Model file for the job. Use its own axes, mm. A direction names the side the tool comes from. Give positions to 0.01 mm unless a question says otherwise; leave off trailing zeros. Loops run counter-clockwise (first coordinate to the right, second up) from the corner with the lowest first, then second, coordinate; pieces in that order, holes last. Notation, with made-up numbers: M 57,-25.5 L 86,-25.5 A28 ccw 86,-0.5 Z; hole C 13,72.5 d8. An arc over 180 degrees is marked long. Answer in a Markdown table with one row per item.
Autodesk Inventor part; units mm, degrees
ref_plane "YZ Plane" through (0, 0, 0) normal (1, 0, 0) x (0, 1, 0)
ref_plane "XZ Plane" through (0, 0, 0) normal (0, 1, 0) x (-1, 0, 0)
ref_plane "XY Plane" through (0, 0, 0) normal (0, 0, 1) x (1, 0, 0)
sketch "Szkic10" plane through (0, 0, 0) normal (0, 1, 0) x (-1, 0, 0)
  line L0 (-25, 60) -> (25, 60)
  line L1 (25, 60) -> (25, -60)
  line L2 (25, -60) -> (-25, -60)
  line L3 (-25, -60) -> (-25, 60)
  line L4 (-25, 60) -> (25, -60) construction
  line L5 (25, 60) -> (-25, -60) construction
  point P0 (0, 0)
  dimension "d75" = 50
  dimension "d76" = 120
extrude "Wyciągnięcie proste6" add sketch "Szkic10" along normal blind 10
sketch "Szkic11" plane through (-25, 0, -60) normal (-1, 0, 0) x (0, 0, 1)
  line L0 (120, 0) -> (0, 0)
  line L1 (120, 0) -> (120, 10)
  line L2 (0, 10) -> (120, 10)
  line L3 (0, 0) -> (0, 10)
  line L4 (0, 0) -> (120, 0)
  line L5 (0, 0) -> (0, 5)
  line L6 (0, 5) -> (120, 5)
  line L7 (0, 5) -> (20, 5)
  line L8 (20, 5) -> (40, 5)
  line L9 (40, 5) -> (80, 5)
  line L10 (80, 5) -> (100, 5)
  circle A0 centre (20, 5) radius 2.5
  circle A1 centre (40, 5) radius 2.5
  circle A2 centre (80, 5) radius 2.5
  circle A3 centre (100, 5) radius 2.5
  point P0 (60, 0)
  dimension "d79" = 5
  dimension "d80" = 20
  dimension "d81" = 20
  dimension "d84" = 5
  dimension "d85" = 5
  dimension "d86" = 5
  dimension "d87" = 5
  dimension "d105" = 20
  dimension "d106" = 20
extrude "Wyciągnięcie proste7" cut sketch "Szkic11" against normal blind 20 contours A3 L6 | L6 A3 | A0 L6 | L6 A0 | A2 L6 | L6 A2 | A1 L6 | L6 A1
sketch "Szkic12" plane through (0, 10, 0) normal (0, 1, 0) x (1, 0, 0)
  line L0 (25, -60) -> (25, 60)
  line L1 (25, 0) -> (3, 0)
  circle A0 centre (3, 0) radius 13
  point P0 (0, 0)
  dimension "d102" = 22
  dimension "d103" = 26
extrude "Wyciągnięcie proste8" cut sketch "Szkic12" against normal up to next
sketch "Szkic13" plane through (0, 0, 0) normal (0, -1, 0) x (1, 0, 0)
  line L0 (25, 60) -> (-25, 60)
  line L1 (-25, 60) -> (-25, -60)
  line L2 (-25, -60) -> (25, -60)
  line L3 (25, -60) -> (25, 60)
  line L4 (25, 60) -> (25, 50)
  line L5 (25, -60) -> (25, 60)
  line L6 (25, 50) -> (-25, 50)
  line L7 (25, -60) -> (25, -50)
  line L8 (25, -50) -> (-25, -50)
  line L9 (25, 50) -> (15, 50)
  line L10 (25, -50) -> (15, -50)
  circle A0 centre (15, 50) radius 5
  circle A1 centre (15, -50) radius 5
  point P0 (0, 0)
  dimension "d93" = 10
  dimension "d94" = 10
  dimension "d95" = 10
  dimension "d96" = 10
  dimension "d97" = 10
  dimension "d98" = 10
extrude "Wyciągnięcie proste9" cut sketch "Szkic13" against normal blind 3 contours A0 L6 | L6 A0 | A1 L8 | L8 A1
sketch "Szkic14" plane through (15, 3, -50) normal (0, -1, 0) x (1, 0, 0)
  circle A0 centre (0, 0) radius 5
  circle A1 centre (0, 100) radius 5
  point P0 (-15, 50)
extrude "Wyciągnięcie proste10" cut sketch "Szkic14" against normal blind 10
sketch "Szkic15" plane through (25, 0, 60) normal (1, 0, 0) x (0, 0, -1)
  line L0 (120, 0) -> (0, 0)
  line L1 (120, 0) -> (120, 10)
  line L2 (0, 10) -> (120, 10)
  line L3 (0, 0) -> (0, 10)
  point P0 (60, 0)
extrude "Wyciągnięcie proste11" add sketch "Szkic15" along normal blind 7
sketch "Szkic16" plane through (-25, 0, 60) normal (0, 0, 1) x (1, 0, 0)
  line L0 (57, 0) -> (0, 0)
  line L1 (57, 10) -> (57, 0)
  line L2 (0, 10) -> (57, 10)
  line L3 (0, 0) -> (0, 10)
  line L4 (35, 10) -> (45, 10)
  line L5 (45, 0) -> (35, 0)
  line L6 (53, 0) -> (45, 0)
  line L7 (57, 0) -> (0, 0)
  line L8 (45, 0) -> (45, 10)
  line L9 (0, 10) -> (57, 10)
  line L10 (57, 10) -> (57, 0)
  line L11 (53, 5) -> (45, 5)
  line L12 (45, 5) -> (49, 5)
  circle A0 centre (49, 5) radius 2
  line L13 (49, 5) -> (53, 5)
  line L14 (53, 5) -> (53, 10)
  line L15 (53, 5) -> (53, 0)
  point P0 (25, 0)
  dimension "d113" = 4
  dimension "d114" = 4
  dimension "d115" = 5
  dimension "d116" = 45
  dimension "d117" = 4
sketch "Szkic17" plane through (-25, 0, -60) normal (0, 0, -1) x (-1, 0, 0)
  line L0 (-53, 10) -> (0, 10)
  line L1 (-53, 0) -> (-53, 10)
  line L2 (0, 0) -> (-53, 0)
  line L3 (0, 10) -> (0, 0)
  line L4 (-35, 0) -> (-45, 0)
  line L5 (-45, 10) -> (-35, 10)
  line L6 (-53, 10) -> (-45, 10)
  line L7 (-53, 10) -> (0, 10)
  line L8 (-45, 10) -> (-45, 0)
  line L9 (0, 0) -> (-53, 0)
  line L10 (-53, 0) -> (-53, 10)
  line L11 (-53, 5) -> (-45, 5)
  line L12 (-45, 5) -> (-49, 5)
  circle A0 centre (-49, 5) radius 2
  line L13 (-49, 5) -> (-53, 5)
  line L14 (-53, 5) -> (-53, 0)
  line L15 (-53, 5) -> (-53, 10)
  line L16 (0, 0) -> (-57, 0)
  line L17 (0, 0) -> (0, 10)
  point P0 (-25, 0)
  point P1 (-25, 10)
  dimension "d119" = 4
  dimension "d120" = 4
  dimension "d121" = 5
  dimension "d122" = 45
  dimension "d123" = 4
hole "Otwór4" at (24, 5, -60) direction (0, 0, 1) diameter 4 depth 20 tip angle 118
hole "Otwór5" at (24, 5, 60) direction (0, 0, -1) diameter 4 depth 20 tip angle 118
sketch "Szkic18" plane through (0, 0, 0) normal (0, -1, 0) x (1, 0, 0)
  circle A0 centre (15, -50) radius 5
  circle A1 centre (15, 50) radius 5
  circle A2 centre (3, 0) radius 13
  line L0 (32, 60) -> (-25, 60)
  line L1 (-25, 60) -> (-25, -60)
  line L2 (-25, -60) -> (32, -60)
  line L3 (32, 60) -> (32, -60)
  line L4 (15, -50) -> (32, -50)
  line L5 (15, 50) -> (32, 50)
  line L6 (32, -60) -> (32, 60)
  line L7 (15, 50) -> (15, 51.5)
  line L8 (15, 51.5) -> (32, 51.5)
  line L9 (15, 50) -> (15, 48.5)
  line L10 (15, 48.5) -> (32, 48.5)
  line L11 (15, -50) -> (15, -48.5)
  line L12 (15, -48.5) -> (32, -48.5)
  line L13 (15, -50) -> (15, -51.5)
  line L14 (15, -51.5) -> (32, -51.5)
  point P0 (0, 0)
  dimension "d138" = 1.5
  dimension "d139" = 1.5
  dimension "d140" = 1.5
  dimension "d141" = 1.5
extrude "Wyciągnięcie proste12" cut sketch "Szkic18" against normal up to next contours L4 L11 L12 A0 | L4 L3 L14 A0 | A0 L14 L13 L4 | A0 L12 L3 L4 | L10 A1 L5 L3 | L5 A1 L8 L3 | L10 L9 L5 A1 | L5 L7 L8 A1
thread "Gwint9"
thread "Gwint10"
thread "Gwint11"
thread "Gwint12"
sketch "Szkic20" plane through (0, 0, 0) normal (0, -1, 0) x (1, 0, 0)
  line L0 (32, 48.5) -> (32, -48.5)
  line L1 (-25, 60) -> (-25, -60)
  circle A0 centre (3, 0) radius 13
  circle A1 centre (22, 16) radius 2.5
  circle A2 centre (22, -16) radius 2.5
  circle A3 centre (-18.5, 0) radius 2.5
  circle A4 centre (3, 0) radius 15
  line L2 (-25, 25) -> (-25, -25)
  line L3 (-25, -25) -> (32, -25)
  line L4 (32, -25) -> (32, 25)
  line L5 (32, 25) -> (-25, 25)
  point P0 (0, 0)
extrude "Wyciągnięcie proste14" cut sketch "Szkic20" against normal up to next contours A1 | A2 | A3
thread "Gwint13"
thread "Gwint14"
thread "Gwint15"
sketch "Szkic21" plane through (0, 10, 0) normal (0, 1, 0) x (1, 0, 0)
  line L0 (32, 48.5) -> (32, -48.5)
  line L1 (32, -51.5) -> (32, -60)
  line L2 (32, 60) -> (32, 30)
  line L3 (-25, -60) -> (-25, 60)
  line L4 (-25, -60) -> (32, -60)
  line L5 (-25, 60) -> (32, 60)
  circle A0 centre (0, 50) radius 2.5
  circle A1 centre (-20, 30) radius 2.5
  circle A2 centre (-20, -30) radius 2.5
  circle A3 centre (0, -50) radius 2.5
  line L6 (-25, -60) -> (32, -60)
  line L7 (32, -51.5) -> (32, -60)
  point P0 (0, 0)
extrude "Wyciągnięcie proste15" cut sketch "Szkic21" against normal up to next
thread "Gwint16"
thread "Gwint17"
thread "Gwint18"
thread "Gwint19"
properties part number "Podstawa górna osi Z"
Q1. Drop flat-ended pins along their axis: pin 1 (2.5 mm diameter, centred on x = 24, y = 5, fed in from +Z); pin 2 (3.5 mm diameter, centred on x = 24, y = 5, fed in from +Z); pin 3 (2.5 mm diameter, centred on y = 5, z = 39, fed in from -X); pin 4 (4.5 mm diameter, centred on x = -18.5, z = 0, fed in from -Y). Give the stop position or say it passes through.
Reported:
| item | result |
|---|---|
| pin 1 | z = 39.55 |
| pin 2 | z = 39.85 |
| pin 3 | x = -5 |
| pin 4 | through |
Q2. 3-axis set-ups, long thin cutter, end or side, ignore diameter. For faces 1 (the face through (3, 5, 60)), 2 (the face through (22.648, 6.474, 44.19)), 3 (the face through (24, 3, -44)), 4 (the face through (-5, 5, 20)), 5 (the face through (26, 4, -48.5)): which of +Z, -Z, +X, -X, +Y, -Y reach the whole face in a straight line?
Reported:
| item | result |
|---|---|
| face 1 | +Z, +X, -X, +Y, -Y |
| face 2 | +Z |
| face 3 | -Z |
| face 4 | -X |
| face 5 | +X, +Y, -Y |
Q3. Saw through at A-A (z = 30). Give the cut face in (x, y), and give its area (3 significant figures).
Reported:
| item | result |
|---|---|
| outline | M -25,0 L -22.5,0 L -22.5,10 L -25,10 Z; M -17.5,0 L 32,0 L 32,10 L -17.5,10 Z |
| area | 520 mm² |
Q4. Probe probe 1 along Z at (x, y) = (22, 2.5); probe 2 along Y at (x, z) = (-19.75, -20); probe 3 along Z at (x, y) = (29, 9.25). List the from-to ranges inside material, lowest first.
Reported:
| item | result |
|---|---|
| probe 1 | -60 to -51.5, -48.5 to -18.5, -13.5 to 13.5, 18.5 to 48.5, 51.5 to 60 |
| probe 2 | 0 to 2.5, 7.5 to 10 |
| probe 3 | -60 to -51.5, -48.5 to 48.5, 51.5 to 60 |
Q5. Saw through at D-D (z = 50). Give the cut face in (x, y).
Reported:
| item | result |
|---|---|
| outline | M -25,0 L -2.5,0 L -2.5,10 L -25,10 Z; M 2.5,0 L 10,0 L 10,10 L 2.5,10 Z |
Q6. Mould opens along X. For faces 6 (the face through (-5, 5, -40)), 7 (the face through (3, 5, -60)), 8 (the face through (24.235, 4.744, -39.007)) say: released by +X, released by -X, zero draft, split by the parting line, or undercut.
Reported:
| item | result |
|---|---|
| face 6 | released by -X |
| face 7 | zero draft |
| face 8 | undercut |
Q7. Saw through at B-B (x = -7). Give the cut face in (y, z).
Reported:
| item | result |
|---|---|
| outline | M 0,-60 L 10,-60 L 10,-8.31 L 0,-8.31 Z; M 0,8.31 L 10,8.31 L 10,60 L 0,60 Z; hole C 5,-40 d5; hole C 5,-20 d5; hole C 5,20 d5; hole C 5,40 d5 |
Q8. Saw through at C-C (x = 0). Give the cut face in (y, z), and give its area (3 significant figures).
Reported:
| item | result |
|---|---|
| outline | M 0,-60 L 10,-60 L 10,-52.5 L 0,-52.5 Z; M 0,-47.5 L 10,-47.5 L 10,-12.65 L 0,-12.65 Z; M 0,12.65 L 10,12.65 L 10,47.5 L 0,47.5 Z; M 0,52.5 L 10,52.5 L 10,60 L 0,60 Z |
| area | 847 mm² |
